Input: dimensioned drawing with shaded views. Units: mm. Origin: part minimum x, y, z. A direction names the side the tool comes from. Round coordinates to 2 decimals unless told otherwise and drop trailing zeros. Write each loop counter-clockwise with the first axis right and the second up, starting at its lowest first coordinate (ties: lowest second). Pieces come first, ordered by that corner, then holes. Notation, with made-up numbers: M 73.25,-37.75 L 77.25,-37.75 A22 ccw 77.25,-4.75 Z; hole C -19.5,73 d9. An arc over 180 degrees is marked long. Answer in a Markdown table with one row per item. Add a question column.
Item 1: Set-up query: the marked faces 1, 2 and 3. Return all of +Z, -Z, +X, -X, +Y, -Y with unobstructed straight access to the full face (end or side cutting, diameter ignored); none if empty.
Item 2: Cut plane D-D on x = 10.75. Return loops of the section in (y, z) (3 decimals).
Item 3: Contact query for flat-ended pins moving along their axis: pin 1 (6 mm diameter, centred on y = 6, z = 8.5, fed in from -X); pin 2 (0.6 mm diameter, centred on y = 1.5, z = 11.5, fed in from +X); pin 3 (7 mm diameter, centred on x = 6, z = 15, fed in from +Y) (3 decimals); pin 4 (1.5 mm diameter, centred on x = 12.5, y = 3.5, fed in from -Z). Output: stop coordinate, or through.
Item 4: Cut plane C-C on z = 6. Return loops of the section in (x, y) (3 decimals), and give its area (3 significant figures).
Item 5: Material intervals for probe 1 along Y at (x, z) = (16.94, 1.2) (3 decimals); probe 2 along X at (y, z) = (4.5, 4); probe 3 along Z at (x, y) = (20.5, 4.25), sorted ascending.
Item 6: Mould query, pull axis X, two halves, no side actions, for the marked faces 4, 5, 6 and 7. Classes: released by +X, released by -X, zero draft, split by the parting line, or undercut.
Item 7: Cut plane B-B on y = 1.5. Return loops of the section in (x, z), and give its area (3 significant figures).
Item 8: Cut plane A-A on x = 16.94. Return loops of the section in (y, z) (3 decimals).
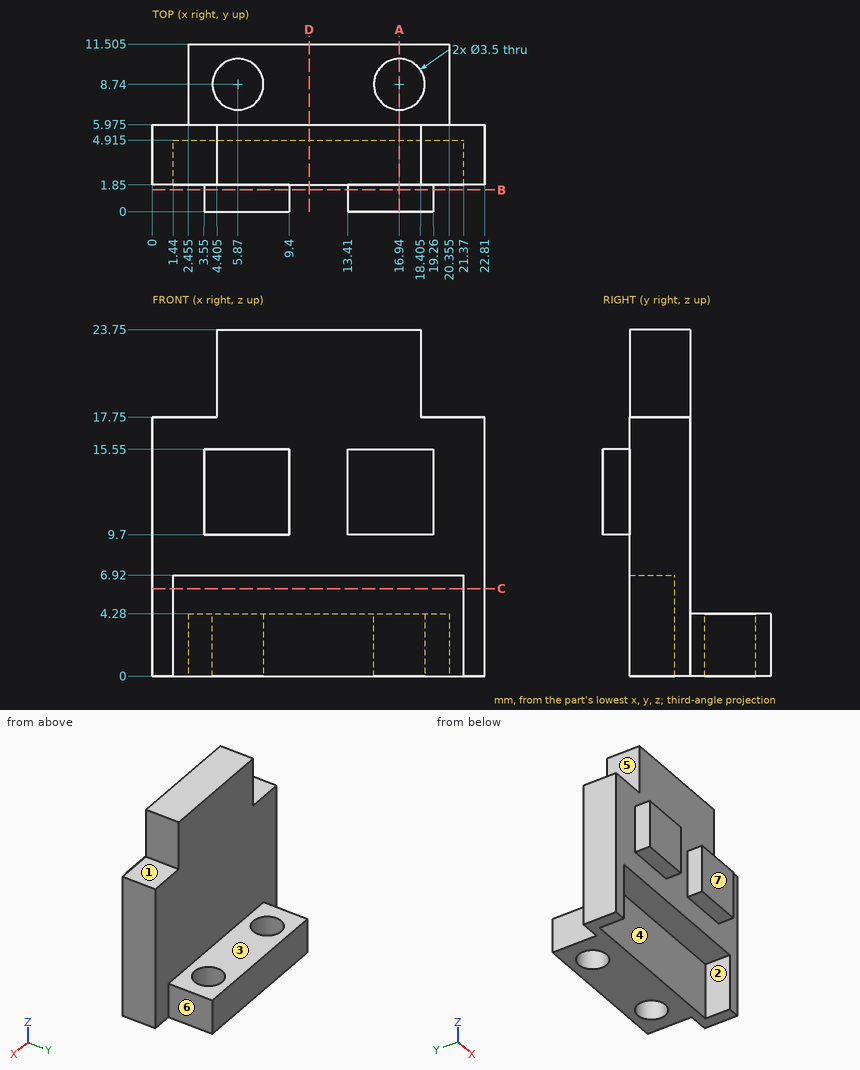
Results below:
| question | item | result |
|---|---|---|
| 1 | face 1 | +Z, +X, +Y, -Y |
| 1 | face 2 | -Z, -Y |
| 1 | face 3 | +Z, +X, -X, +Y |
| 2 | outline | M 1.85,6.92 L 4.915,6.92 L 4.915,0 L 11.505,0 L 11.505,4.28 L 5.975,4.28 L 5.975,23.75 L 1.85,23.75 Z |
| 3 | pin 1 | x = 0 |
| 3 | pin 2 | x = 19.26 |
| 3 | pin 3 | y = 5.975 |
| 3 | pin 4 | z = 6.92 |
| 4 | outline | M 0,1.85 L 1.44,1.85 L 1.44,4.915 L 21.37,4.915 L 21.37,1.85 L 22.81,1.85 L 22.81,5.975 L 0,5.975 Z |
| 4 | area | 33.0 mm2 |
| 5 | probe 1 | 4.915 to 6.99, 10.49 to 11.505 |
| 5 | probe 2 | 0 to 1.44, 21.37 to 22.81 |
| 5 | probe 3 | 6.92 to 17.75 |
| 6 | face 4 | undercut |
| 6 | face 5 | released by -X |
| 6 | face 6 | released by +X |
| 6 | face 7 | zero draft |
| 7 | outline | M 3.55,9.7 L 9.4,9.7 L 9.4,15.55 L 3.55,15.55 Z; M 13.41,9.7 L 19.26,9.7 L 19.26,15.55 L 13.41,15.55 Z |
| 7 | area | 68.4 mm2 |
| 8 | outline | M 0,9.7 L 1.85,9.7 L 1.85,6.92 L 4.915,6.92 L 4.915,0 L 6.99,0 L 6.99,4.28 L 5.975,4.28 L 5.975,23.75 L 1.85,23.75 L 1.85,15.55 L 0,15.55 Z; M 10.49,0 L 11.505,0 L 11.505,4.28 L 10.49,4.28 Z |
